Check sheet for the modelled part. Datum: model origin and axes. Units: mm. Round coordinates to 2 decimals unless told otherwise and drop trailing zeros. Write each loop counter-clockwise with the first axis right and the second up, starting at its lowest first coordinate (ties: lowest second). Pieces come first, ordered by that corner, then holes. Notation, with made-up numbers: (83.5, 3.25) -> (128.5, 3.25) arc R34 ccw to (128.5, 36.25) -> close; hole circle Ø10 at (52, 42). An arc over 180 degrees is marked (long way). Put each result on its own line as item: value. Start each with the question number.
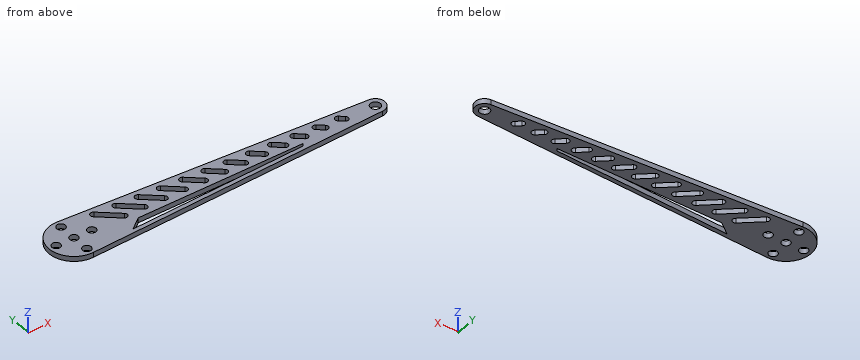
from build123d import *

# Parameters (mm, degrees)
SKETCH_2_R      = 1.7
SKETCH_2_R_2    = 2
EXTRUDE_1_DEPTH = 2


with BuildPart() as part:
    # 草图2 → 凸台-拉伸1 (new body)
    with BuildSketch(Plane.XY):
        with BuildLine():
            Line((120.1953125, 3.744910283), (0.520833333, 9.986427421))
            ThreePointArc((0.520833333, 9.986427421), (-10, 0), (0.520833333, -9.986427421))
            Line((0.520833333, -9.986427421), (120.1953125, -3.744910283))
            ThreePointArc((120.1953125, -3.744910283), (123.75, 0), (120.1953125, 3.744910283))
        make_face()
        with Locations((0, 7.1)):
            Circle(SKETCH_2_R, mode=Mode.SUBTRACT)
        Circle(SKETCH_2_R, mode=Mode.SUBTRACT)
        with Locations((7.1, 0)):
            Circle(SKETCH_2_R, mode=Mode.SUBTRACT)
        with Locations((-7.1, 0)):
            Circle(SKETCH_2_R, mode=Mode.SUBTRACT)
        with Locations((0, -7.1)):
            Circle(SKETCH_2_R, mode=Mode.SUBTRACT)
        with Locations((120, 0)):
            Circle(SKETCH_2_R_2, mode=Mode.SUBTRACT)
        with BuildLine():
            Line((19.199560495, -0.96370295), (11.58500645, 5.399602936))
            ThreePointArc((11.58500645, 5.399602936), (11.426647663, 7.168650049), (13.195694776, 7.327008836))
            Line((13.195694776, 7.327008836), (20.810248822, 0.96370295))
            ThreePointArc((20.810248822, 0.96370295), (20.968607609, -0.805344163), (19.199560495, -0.96370295))
        make_face(mode=Mode.SUBTRACT)
        with BuildLine():
            Line((27.198443723, -0.959170233), (20.116072333, 4.959402974))
            ThreePointArc((20.116072333, 4.959402974), (19.958458377, 6.720129483), (21.719184886, 6.87774344))
            Line((21.719184886, 6.87774344), (28.801556277, 0.959170233))
            ThreePointArc((28.801556277, 0.959170233), (28.959170233, -0.801556277), (27.198443723, -0.959170233))
        make_face(mode=Mode.SUBTRACT)
        with BuildLine():
            Line((35.198443723, -0.959170233), (28.64858146, 4.51439747))
            ThreePointArc((28.64858146, 4.51439747), (28.490967504, 6.275123979), (30.251694013, 6.432737935))
            Line((30.251694013, 6.432737935), (36.801556277, 0.959170233))
            ThreePointArc((36.801556277, 0.959170233), (36.959170233, -0.801556277), (35.198443723, -0.959170233))
        make_face(mode=Mode.SUBTRACT)
        with BuildLine():
            Line((43.198443723, -0.959170233), (37.181090587, 4.069391965))
            ThreePointArc((37.181090587, 4.069391965), (37.023476631, 5.830118475), (38.784203141, 5.987732431))
            Line((38.784203141, 5.987732431), (44.801556277, 0.959170233))
            ThreePointArc((44.801556277, 0.959170233), (44.959170233, -0.801556277), (43.198443723, -0.959170233))
        make_face(mode=Mode.SUBTRACT)
        with BuildLine():
            Line((51.198443723, -0.959170233), (45.713599714, 3.624386461))
            ThreePointArc((45.713599714, 3.624386461), (45.555985758, 5.38511297), (47.316712268, 5.542726927))
            Line((47.316712268, 5.542726927), (52.801556277, 0.959170233))
            ThreePointArc((52.801556277, 0.959170233), (52.959170233, -0.801556277), (51.198443723, -0.959170233))
        make_face(mode=Mode.SUBTRACT)
        with BuildLine():
            Line((59.198443723, -0.959170233), (54.246108842, 3.179380957))
            ThreePointArc((54.246108842, 3.179380957), (54.088494885, 4.940107466), (55.849221395, 5.097721422))
            Line((55.849221395, 5.097721422), (60.801556277, 0.959170233))
            ThreePointArc((60.801556277, 0.959170233), (60.959170233, -0.801556277), (59.198443723, -0.959170233))
        make_face(mode=Mode.SUBTRACT)
        with BuildLine():
            Line((67.198443723, -0.959170233), (62.778617969, 2.734375453))
            ThreePointArc((62.778617969, 2.734375453), (62.621004012, 4.495101962), (64.381730522, 4.652715918))
            Line((64.381730522, 4.652715918), (68.801556277, 0.959170233))
            ThreePointArc((68.801556277, 0.959170233), (68.959170233, -0.801556277), (67.198443723, -0.959170233))
        make_face(mode=Mode.SUBTRACT)
        with BuildLine():
            Line((75.198443723, -0.959170233), (71.311127096, 2.289369948))
            ThreePointArc((71.311127096, 2.289369948), (71.153513139, 4.050096458), (72.914239649, 4.207710414))
            Line((72.914239649, 4.207710414), (76.801556277, 0.959170233))
            ThreePointArc((76.801556277, 0.959170233), (76.959170233, -0.801556277), (75.198443723, -0.959170233))
        make_face(mode=Mode.SUBTRACT)
        with BuildLine():
            Line((83.198443723, -0.959170233), (79.843636223, 1.844364444))
            ThreePointArc((79.843636223, 1.844364444), (79.686022267, 3.605090953), (81.446748776, 3.76270491))
            Line((81.446748776, 3.76270491), (84.801556277, 0.959170233))
            ThreePointArc((84.801556277, 0.959170233), (84.959170233, -0.801556277), (83.198443723, -0.959170233))
        make_face(mode=Mode.SUBTRACT)
        with BuildLine():
            Line((91.198443723, -0.959170233), (88.37614535, 1.39935894))
            ThreePointArc((88.37614535, 1.39935894), (88.218531394, 3.160085449), (89.979257903, 3.317699405))
            Line((89.979257903, 3.317699405), (92.801556277, 0.959170233))
            ThreePointArc((92.801556277, 0.959170233), (92.959170233, -0.801556277), (91.198443723, -0.959170233))
        make_face(mode=Mode.SUBTRACT)
        with BuildLine():
            Line((99.198443723, -0.959170233), (96.908654477, 0.954353436))
            ThreePointArc((96.908654477, 0.954353436), (96.751040521, 2.715079945), (98.51176703, 2.872693901))
            Line((98.51176703, 2.872693901), (100.801556277, 0.959170233))
            ThreePointArc((100.801556277, 0.959170233), (100.959170233, -0.801556277), (99.198443723, -0.959170233))
        make_face(mode=Mode.SUBTRACT)
        with BuildLine():
            Line((107.198443723, -0.959170233), (105.441163604, 0.509347931))
            ThreePointArc((105.441163604, 0.509347931), (105.283549648, 2.270074441), (107.044276157, 2.427688397))
            Line((107.044276157, 2.427688397), (108.801556277, 0.959170233))
            ThreePointArc((108.801556277, 0.959170233), (108.959170233, -0.801556277), (107.198443723, -0.959170233))
        make_face(mode=Mode.SUBTRACT)
        Polygon((22.985742471, -3.574018318), (89.177701626, -2.685452731), (88.37614535, -3.744910283), (18.132146509, -7.408424222), align=None, mode=Mode.SUBTRACT)
    extrude(amount=EXTRUDE_1_DEPTH)


solid = part.part
1. Section check B-B, the plane x = 58. Enter the section's corners in (y, z), then the cut area to 3 significant figures.
2. Material ranges on L1, parallel to Y at x = 0, z = 0.4; L2, parallel to Y at x = 52, z = 1.55; L3, parallel to Y at x = 120, z = 1.05, recorded low to high. Write a range as [from, to].
3. Section check C-C, the plane z = 1.35. Give the number of separate pieces and of enclosed holes in the cut face, then the cut area to 3 significant figures.
4. Section check A-A, the plane x = -7.1. Enter the section's corners in (y, z), then the cut area to 3 significant figures.
5. Gauge pin test, flat end, axial feed: P1, Ø6.5, axis at x = 120, y = 0, coming from the -Z side. Record the tip position at first contact, or that the pin passes through.
6. Section check D-D, the plane x = 7.1. Enter the section's corners in (y, z), then the cut area to 3 significant figures.
Reply:
1. outline: (-6.99, 0) -> (-5.33, 0) -> (-5.33, 2) -> (-6.99, 2) -> close; (-3.1, 0) -> (0.04, 0) -> (0.04, 2) -> (-3.1, 2) -> close; (3.3, 0) -> (6.99, 0) -> (6.99, 2) -> (3.3, 2) -> close
1. area: 17.0 mm2
2. L1: y = [-10, -8.8], [-5.4, -1.7], [1.7, 5.4], [8.8, 10]
2. L2: y = [-7.3, -5.64], [-3.18, -1.25], [1.63, 7.3]
2. L3: y = [-3.76, -2], [2, 3.76]
3. separate pieces: 1
3. enclosed holes: 19
3. area: 1,370 mm2
4. outline: (-7.04, 0) -> (-1.7, 0) -> (-1.7, 2) -> (-7.04, 2) -> close; (1.7, 0) -> (7.04, 0) -> (7.04, 2) -> (1.7, 2) -> close
4. area: 21.4 mm2
5. P1: stops at z = 0
6. outline: (-9.64, 0) -> (-1.7, 0) -> (-1.7, 2) -> (-9.64, 2) -> close; (1.7, 0) -> (9.64, 0) -> (9.64, 2) -> (1.7, 2) -> close
6. area: 31.8 mm2
